Geometry: final body of the model. Coordinates: model frame, mm. Give positions to 0.01 mm unless a question says otherwise; leave off trailing zeros. Order: outer loops, then holes, each group sorted by start corner. A loop starts at its lowest first (then second) coordinate and runs counter-clockwise, first axis right, second up. Notation, with made-up numbers: (4, -19) -> (56, -19) arc R10 cw to (56, -1) -> close; hole circle Ø8 at (-18.5, -24). An arc over 180 degrees is marked (long way). One line per question, with ' | ' between items.
from build123d import *

# Parameters (mm, degrees)
F1_DEPTH = 3
F2_R     = 4.99999


# Not quite as in the source:
# - a fillet or chamfer is up to 0.001 mm smaller than in the source, because OpenCascade refuses the exact size


with BuildPart() as f1:
    # F0 (on Front) → F1 (new body)
    with BuildSketch(Plane.XZ):
        Polygon((80.6066017178, 0), (0, 0), (0, -10.6066017178), (70, -10.6066017178), (70, -40.6066017178), (10, -40.6066017178), (10, -51.2132034356), (49.3933982822, -51.2132034356), (49.3933982822, -111.8198051534), (76.5, -111.8198051534), (76.5, -101.2132034356), (71.5, -101.2132034356), (71.5, -108.2132034356), (68.5, -108.2132034356), (68.5, -101.2132034356), (60, -101.2132034356), (60, -51.2132034356), (80.6066017178, -51.2132034356), align=None)
    extrude(amount=F1_DEPTH)

    # F2 (radius 5 in the source; OpenCascade refuses exactly that, so slightly less here)
    f2_edges = [f1.edges().sort_by_distance(p)[0] for p in [
        (49.393398, -1.5, -51.213203),
        (70, -1.5, -10.606602),
        (70, -1.5, -40.606602),
        (80.606602, -1.5, 0),
        (80.606602, -1.5, -51.213203),
        (60, -1.5, -51.213203),
        (60, -1.5, -101.213203),
        (76.5, -1.5, -101.213203),
        (76.5, -1.5, -111.819805),
        (49.393398, -1.5, -111.819805),
    ]]
    fillet(f2_edges, radius=F2_R)


solid = f1.part
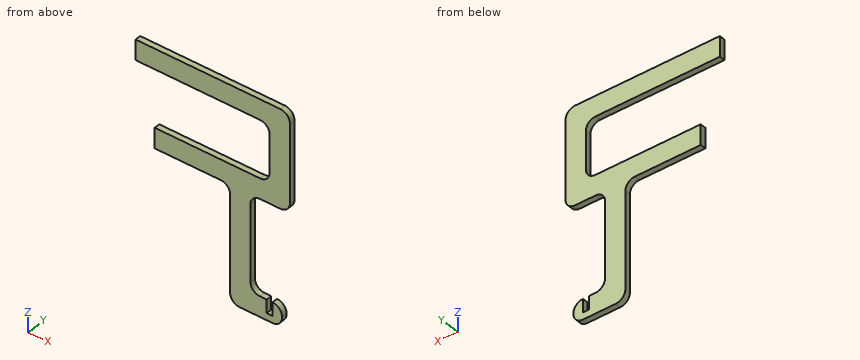
1) Section A-A on x = 31. Return loops of the section in (y, z).
Check result:
outline: (-3, -51.21) -> (0, -51.21) -> (0, -40.61) -> (-3, -40.61) -> close; (-3, -10.61) -> (0, -10.61) -> (0, 0) -> (-3, 0) -> close
2) Section B-B on x = 62.5. Return loops of the section in (y, z), plus the area to 3 significant figures.
Check result:
outline: (-3, -111.82) -> (0, -111.82) -> (0, -100.54) -> (-3, -100.54) -> close; (-3, -51.88) -> (0, -51.88) -> (0, -40.61) -> (-3, -40.61) -> close; (-3, -10.61) -> (0, -10.61) -> (0, 0) -> (-3, 0) -> close | area: 99.5 mm^2
3) Material intervals for probe 1 along Z at (x, y) = (33, -0.65); probe 2 along Z at (x, y) = (55, -0.4); probe 3 along Z at (x, y) = (69.5, -1.55), sorted ascending. Write a range as from..to.
Check result:
probe 1: z = -51.21..-40.61, -10.61..0 | probe 2: z = -111.82..-40.61, -10.61..0 | probe 3: z = -111.82..-108.21, -51.21..-37.79, -13.43..0
4) Contact query for flat-ended pins moving along their axis: pin 1 Ø0.9 at (y, z) = (-2, -46.5) entering from -X; pin 2 Ø0.9 at (y, z) = (-1.5, -104) entering from -X; pin 3 Ø0.9 at (x, y) = (32, -1.5) entering from -Z. Output: stop coordinate, or through.
Check result:
pin 1: stops at x = 10 | pin 2: stops at x = 49.39 | pin 3: stops at z = -51.21
5) Section D-D on z = -22. Return loops of the section in (x, y).
Check result:
outline: (70, -3) -> (80.61, -3) -> (80.61, 0) -> (70, 0) -> close
